Part model, mm, in its own coordinate system. A direction names the side the tool comes from. Give positions to 0.01 mm unless a question says otherwise; leave off trailing zeros. Order: outer loops, then holes, each group sorted by start corner. A loop starts at its lowest first (then second) coordinate and runs counter-clockwise, first axis right, second up. Notation, with made-up numbers: M 49,-4.5 L 86,-4.5 A27 ccw 86,25.5 Z; hole C 68.25,60.25 d1. An arc over 180 degrees is marked long. Answer as a JSON object with one key per item and string values.
from build123d import *

# Parameters (mm, degrees)
F0_W     = 50
F0_H     = 85
F1_DEPTH = 40
F2_W     = 48
F2_H     = 83
F3_DEPTH = 38
F5_DEPTH = 5
F6_R     = 0.75
F7_DEPTH = 5


with BuildPart() as f1:
    # F0 (on Top) → F1 (new body)
    with BuildSketch(Plane.XY):
        with Locations((-9.93821384, -5.5663399398)):
            Rectangle(F0_W, F0_H)
    extrude(amount=F1_DEPTH)

    # F2 (on face) → F3 (cut)
    with BuildSketch(Plane.XY.offset(40)):
        with Locations((-10.0635439157, -5.6413925663)):
            Rectangle(F2_W, F2_H)
    extrude(amount=-F3_DEPTH, mode=Mode.SUBTRACT)

    # F4 (on face) → F5 (join)
    with BuildSketch(Plane.XY.offset(2)):
        with BuildLine():
            Line((-30.0635439157, 31.8586074337), (-30.0635439157, 33.3586074337))
            ThreePointArc((-30.0635439157, 33.3586074337), (-31.1242040875, 32.9192676054), (-31.5635439157, 31.8586074337))
            Line((-31.5635439157, 31.8586074337), (-30.0635439157, 31.8586074337))
        make_face()
        with BuildLine():
            ThreePointArc((-31.5635439157, 31.8586074337), (-30.0635439157, 30.3586074337), (-28.5635439157, 31.8586074337))
            ThreePointArc((-28.5635439157, 31.8586074337), (-29.002883744, 32.9192676054), (-30.0635439157, 33.3586074337))
            Line((-30.0635439157, 33.3586074337), (-30.0635439157, 31.8586074337))
            Line((-30.0635439157, 31.8586074337), (-31.5635439157, 31.8586074337))
        make_face()
    extrude(amount=F5_DEPTH)

    # F6 (on face) → F7 (cut)
    with BuildSketch(Plane.XY.offset(7)):
        with Locations((-30.0635439157, 31.8586074337)):
            Circle(F6_R)
    extrude(amount=-F7_DEPTH, mode=Mode.SUBTRACT)


solid = f1.part
1. Cut at A-A on z = 4. Give the cut face in (x, y), plus the area to 3 significant figures.
Worked answers:
{"outline": "M -34.94,-48.07 L 15.06,-48.07 L 15.06,36.93 L -34.94,36.93 Z; C -30.06,31.86 d3; hole M -34.06,-47.14 L 13.94,-47.14 L 13.94,35.86 L -34.06,35.86 Z; hole C -30.06,31.86 d1.5", "area": "271 mm^2"}
2. Cut at C-C on y = 16. Give the cut face in (x, z), plus the area to 3 significant figures.
Worked answers:
{"outline": "M -34.94,0 L 15.06,0 L 15.06,40 L 13.94,40 L 13.94,2 L -34.06,2 L -34.06,40 L -34.94,40 Z", "area": "176 mm^2"}
3. Probe line 1 along Y through (x, z) = (13, 33.5); line 2 along X through (y, z) = (-24.5, 20.5); line 3 along Z through (x, y) = (-27.5, -36.5). List the from-to ranges inside material, lowest first.
Worked answers:
{"line 1": "y = -48.07 to -47.14, 35.86 to 36.93", "line 2": "x = -34.94 to -34.06, 13.94 to 15.06", "line 3": "z = 0 to 2"}
4. Two-plate mould, pull along X, no slides. Class faces 3 (the flat face through (-10, -5, 0)), 4 (the flat face through (-10, -47.141, 21)), 5 (the flat face through (15.062, -6, 20)): +X half, -X half, draft (parallel to the pull), parting line (faces both ways), or undercut.
Worked answers:
{"face 3": "draft", "face 4": "undercut", "face 5": "+X half"}
5. Which spindle directions (+Z, -Z, +X, -X, +Y, -Y) get a long thin tool onto all of the face, cutting with end or side? Do faces 1 (the flat face through (-10, 35.859, 21)), 2 (the flat face through (-10, 36.934, 20)). Say none if no direction does.
Worked answers:
{"face 1": "+Z", "face 2": "+Z, -Z, +X, -X, +Y"}
6. Cut at D-D on x = 8. Give the cut face in (y, z), plus the area to 3 significant figures.
Worked answers:
{"outline": "M -48.07,0 L 36.93,0 L 36.93,40 L 35.86,40 L 35.86,2 L -47.14,2 L -47.14,40 L -48.07,40 Z", "area": "246 mm^2"}
7. Cut at B-B on z = 13.5. Give the cut face in (x, y), plus the area to 3 significant figures.
Worked answers:
{"outline": "M -34.94,-48.07 L 15.06,-48.07 L 15.06,36.93 L -34.94,36.93 Z; hole M -34.06,-47.14 L 13.94,-47.14 L 13.94,35.86 L -34.06,35.86 Z", "area": "266 mm^2"}
8. Pin check, flat tips, straight feed: P1, Ø6, axis at x = 8, y = 7, coming from the +Z side; P2, Ø3.5, axis at x = -30.5, y = 32.5, coming from the +Z side. Stop position of each tip, or through.
Worked answers:
{"P1": "stops at z = 2", "P2": "stops at z = 7"}
